from build123d import *

# Parameters (mm, degrees)
F1_DEPTH = 63.5
F2_DEPTH = 25.4
F3_DEPTH = 7.9375
F5_R     = 5.08


with BuildPart() as f1:
    # F0 (on Front) → F1 (new body, symmetric)
    with BuildSketch(Plane.XZ):
        Polygon((41.275, -9.525), (41.275, 9.525), (31.3690012749, 9.525), (-41.275, 9.525), (-41.275, -9.525), align=None)
    extrude(amount=F1_DEPTH, both=True)

    # F0 (on Front) → F2 (join, symmetric)
    with BuildSketch(Plane.XZ):
        with BuildLine():
            Line((31.3690012749, 9.525), (41.275, 9.525))
            Line((41.275, 9.525), (41.275, 28.2690877087))
            ThreePointArc((41.275, 28.2690877087), (44.4961665848, 37.8553343621), (52.8524645544, 43.5513262258))
            Line((52.8524645544, 43.5513262258), (69.7987371812, 43.5513262258))
            Line((69.7987371812, 43.5513262258), (69.7987371812, 52.7542612036))
            Line((69.7987371812, 52.7542612036), (50.1708027815, 53.0874418332))
            ThreePointArc((50.1708027815, 53.0874418332), (36.6001755499, 43.837151504), (31.3690012749, 28.2690877087))
            Line((31.3690012749, 28.2690877087), (31.3690012749, 9.525))
        make_face()
        Polygon((69.7987371812, 52.7542612036), (69.7987371812, 43.5513262258), (69.7987371812, 38.1), (101.6512628188, 38.1), (101.6512628188, 66.675), (69.7987371812, 66.675), align=None)
    extrude(amount=F2_DEPTH, both=True)

    # F0 (on Front) → F3 (join, symmetric)
    with BuildSketch(Plane.XZ):
        with BuildLine():
            Line((-41.275, 9.525), (31.3690012749, 9.525))
            Line((31.3690012749, 9.525), (31.3690012749, 28.2690877087))
            ThreePointArc((31.3690012749, 28.2690877087), (36.6001755499, 43.837151504), (50.1708027815, 53.0874418332))
            Line((50.1708027815, 53.0874418332), (69.7987371812, 52.7542612036))
            Line((69.7987371812, 52.7542612036), (69.7987371812, 66.675))
            add(Edge.make_bspline(
                [(0.9200547216, 44.4546873168), (21.9732050528, 57.1926332926), (55.5999299853, 69.1414192126), (66.4309648739, 66.6444715672), (69.7987371812, 66.675)],
                knots=[0.3021299469, 0.3021299469, 0.3021299469, 0.3021299469, 0.7310163448, 1, 1, 1, 1], degree=3))
            add(Edge.make_bspline(
                [(0.9200547224, 44.4546873157), (5.3862455156, 44.3452942524), (7.7617773977, 44.1589559848), (0.6045961391, 44.2634363016)],
                knots=[6.1143383921, 6.1143383921, 6.1143383921, 6.1143383921, 12.0207626888, 12.0207626888, 12.0207626888, 12.0207626888], degree=3))
            add(Edge.make_bspline(
                [(-41.275, 9.525), (-29.0215326785, 23.7296115654), (-14.1237601662, 35.3160902289), (0.6045961391, 44.2634363016)],
                knots=[0, 0, 0, 0, 0.2999880046, 0.2999880046, 0.2999880046, 0.2999880046], degree=3))
        make_face()
    extrude(amount=F3_DEPTH, both=True)

    # F0 (on Front) → F4 (revolve)
    with BuildSketch(Plane.XZ):
        Polygon((69.7987371812, 52.7542612036), (69.7987371812, 43.5513262258), (69.7987371812, 38.1), (101.6512628188, 38.1), (101.6512628188, 66.675), (69.7987371812, 66.675), align=None)
    revolve(axis=Axis((101.6512628188, 0, 52.3875), (0, 0, -1)))

    # F5
    f5_edges = [f1.edges().sort_by_distance(p)[0] for p in [
        (-41.275, -63.5, 0),
        (41.275, -63.5, 0),
        (-41.275, 63.5, 0),
        (41.275, 63.5, 0),
    ]]
    fillet(f5_edges, radius=F5_R)


solid = f1.part
For this review, take the finished solid that the model builds, in its own axes (mm). A direction names the side the tool comes from. Coordinates: 2 decimals unless noted, no trailing zeros. Order: outer loops, then holes, each group sorted by start corner. A loop starts at its lowest first (then second) coordinate and runs counter-clockwise, first axis right, second up. Notation, with made-up numbers: (-14.5, 11) - (3.5, 11) arc R23 cw to (3.5, 35) - close; hole circle Ø2 at (-9, 11). An arc over 180 degrees is marked (long way). Use one line per item in the form item = value.
Q1. For probe 1 along X at (y, z) = (21, 2) (3 decimals); probe 2 along Z at (x, y) = (28, -30) (3 decimals); probe 3 along Y at (x, z) = (74.5, 47.5), list the stretches that pass through material, from the lowest coordinate up. Write a range as from..to.
Checked values:
probe_1 = -41.275..41.275
probe_2 = -9.525..9.525
probe_3 = -25.4..25.4
Q2. Consider section C-C (x = 91). Give the boundary of the cut face in (y, z) (3 decimals).
Checked values:
outline = (-30.019, 38.1) - (30.019, 38.1) - (30.019, 66.675) - (-30.019, 66.675) - close
Q3. Draft analysis for pull direction X (two halves, no side actions). For faces 1 (the cylindrical face through (39.75, -62.05, 0.13)), 2 (the cylindrical face through (-39.75, 62.05, -0.13)), 3 (the flat face through (69.799, 0, 41)), state which applies: +X half, -X half, draft (parallel to the pull), parting line (faces both ways), or undercut.
Checked values:
face_1 = +X half
face_2 = -X half
face_3 = undercut
Q4. For faces 4 (the flat face through (31.369, -17, 19)), 5 (the flat face through (41.275, -1, 5)), 6 (the cylindrical face through (36.74, 16.55, 44.02)), list the 3-axis set-ups (+Z, -Z, +X, -X, +Y, -Y) from which the entire face can be reached by the end or side of a thin tool; tool diameter is ignored.
Checked values:
face_4 = +Z, -X, -Y
face_5 = -Z, +X, +Y, -Y
face_6 = +Z, -X, +Y
Q5. Consider section B-B (y = -55). Give the boundary of the cut face in (x, z) (3 decimals), then the cut area to 3 significant figures.
Checked values:
outline = (-41.275, -9.525) - (41.275, -9.525) - (41.275, 9.525) - (-41.275, 9.525) - close
area = 1,570 mm2
Q6. For P1, Ø6, axis at x = 2, y = 47.5, coming from the +Z side (3 decimals); P2, Ø10, axis at y = -22, z = 56.5, coming from the -X side; P3, Ø4, axis at x = 8.5, z = 51, coming from the -Y side, all flat-tipped, find the tip position at first contact; note any pin that passes through.
Checked values:
P1 = 9.525
P2 = 45.97
P3 = -7.94
Q7. Consider section A-A (z = 0.5). Give the boundary of the cut face in (x, y) (3 decimals).
Checked values:
outline = (-41.275, -58.42) arc R5.08 ccw to (-36.195, -63.5) - (36.195, -63.5) arc R5.08 ccw to (41.275, -58.42) - (41.275, 58.42) arc R5.08 ccw to (36.195, 63.5) - (-36.195, 63.5) arc R5.08 ccw to (-41.275, 58.42) - close
